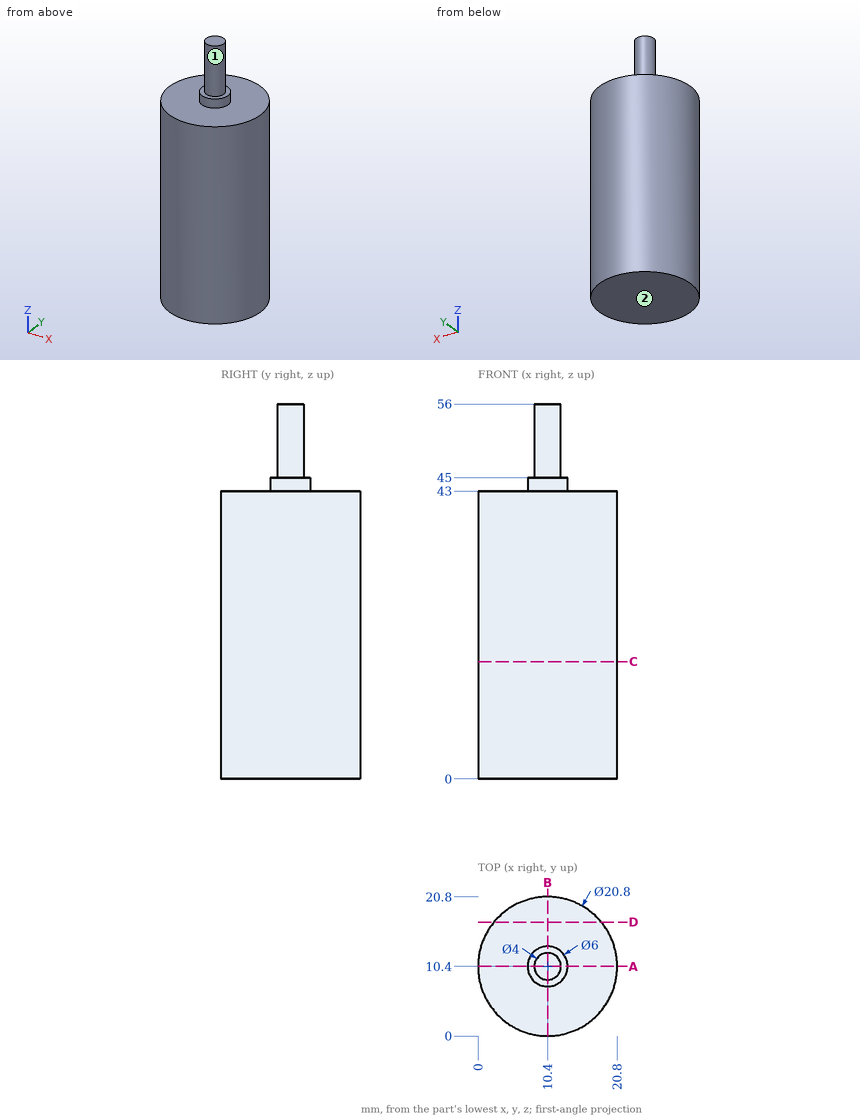
Verification items for this drawing (mm, ordinates from the low corner). A direction names the side the tool comes from. Round coordinates to 2 decimals unless told otherwise and drop trailing zeros. Order: outer loops, then holes, each group sorted by start corner. A loop starts at its lowest first (then second) coordinate and runs counter-clockwise, first axis right, second up. Notation, with made-up numbers: M 57,-23 L 115,-23 A9 cw 115,-19 Z; hole C 56,-19.75 d9. An arc over 180 degrees is marked long. Answer in a Markdown table with one row per item. Add a question column.
Item 1: Material ranges on L1, parallel to Z at x = 10.75, y = 5; L2, parallel to Z at x = 9.25, y = 13; L3, parallel to Y at x = 18, z = 7, recorded low to high. Write a range as [from, to].
Item 2: Set-up check for the marked faces 1 and 2: record each of +Z, -Z, +X, -X, +Y, -Y from which the full face is reachable in a straight line by a thin tool's end or side.
Item 3: Sectioned sample at A-A, the plane y = 10.4. Enter the section's corners in (x, z), plus the area to 3 significant figures.
Item 4: Sectioned sample at C-C, the plane z = 17.5. Enter the section's corners in (x, y).
Item 5: Sectioned sample at D-D, the plane y = 17. Enter the section's corners in (x, z).
Item 6: Depth check by flat-ended pin: pin 1 Ø1 at (y, z) = (3.5, 12) entering from -X; pin 2 Ø2 at (y, z) = (8, 7) entering from +X; pin 3 Ø2 at (x, z) = (18, 8) entering from -Y. Enter the tip coordinate at first touch or a pass-through.
Filled in:
| question | item | result |
|---|---|---|
| 1 | L1 | z = [0, 43] |
| 1 | L2 | z = [0, 45] |
| 1 | L3 | y = [3.3, 17.5] |
| 2 | face 1 | +Z |
| 2 | face 2 | -Z, +X, -X, +Y, -Y |
| 3 | outline | M 0,0 L 20.8,0 L 20.8,43 L 13.4,43 L 13.4,45 L 12.4,45 L 12.4,56 L 8.4,56 L 8.4,45 L 7.4,45 L 7.4,43 L 0,43 Z |
| 3 | area | 950 mm² |
| 4 | outline | C 10.4,10.4 d20.8 |
| 5 | outline | M 2.36,0 L 18.44,0 L 18.44,43 L 2.36,43 Z |
| 6 | pin 1 | stops at x = 2.2 |
| 6 | pin 2 | stops at x = 20.71 |
| 6 | pin 3 | stops at y = 2.36 |
